Geometry check sheet. Reference: the model listing, model coordinates, mm. Face numbers are marked on the shaded views. Give positions to 0.01 mm unless a question says otherwise; leave off trailing zeros. Order: outer loops, then holes, each group sorted by start corner. A loop starts at its lowest first (then second) coordinate and runs counter-clockwise, first axis right, second up.
```python
from build123d import *

# Parameters (mm, degrees)
F1_DEPTH = 8
F2_D     = 15
F3_D     = 15
F5_W     = 30
F5_H     = 4
F6_DEPTH = 30.001


with BuildPart() as f1:
    # F0 (on Front) → F1 (new body)
    with BuildSketch(Plane.XZ):
        with BuildLine():
            Line((110, 15), (0, 15))
            ThreePointArc((0, 15), (-15, 0), (0, -15))
            Line((0, -15), (110, -15))
            ThreePointArc((110, -15), (125, 0), (110, 15))
        make_face()
    extrude(amount=F1_DEPTH)

    # F2 (through all)
    with Locations(Plane(origin=(0, 0, 0), x_dir=(1, 0, 0), z_dir=(0, 1, 0))):
        with Locations((0, 0)):
            Hole(F2_D / 2)

    # F3 (through all)
    with Locations(Plane(origin=(0, 0, 0), x_dir=(1, 0, 0), z_dir=(0, 1, 0))):
        with Locations((110, 0)):
            Hole(F3_D / 2)

    # F5 (on offset) → F6 (cut, through all)
    with BuildSketch(Plane.XY.offset(15)):
        with Locations((0, -4.0625976841)):
            Rectangle(F5_W, F5_H)
    extrude(amount=-F6_DEPTH, mode=Mode.SUBTRACT)


solid = f1.part
```
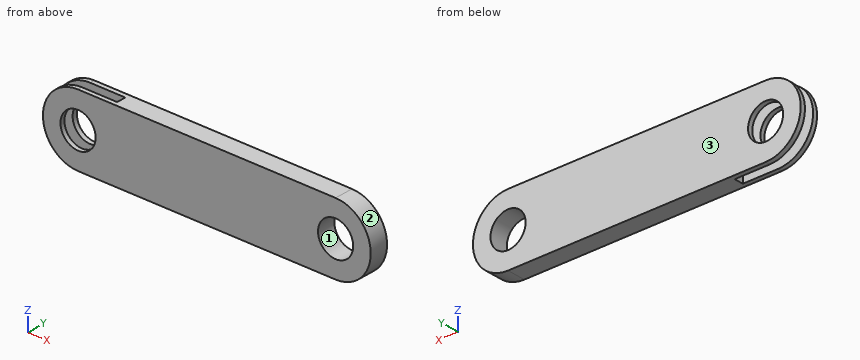
Q1. Gauge pin test, flat ends, axial feed: P1, Ø1.2, axis at y = -4, z = -7, coming from the -X side; P2, Ø9, axis at x = 1.5, z = -2, coming from the +Y side; P3, Ø1, axis at y = -1, z = -8.5, coming from the +X side. Record the tip position at first contact, or that the pin passes through.
Q2. Thickness scan on L1, parallel to Z at x = 110, y = -5.75; L2, parallel to X at y = -7.25, z = -13; L3, parallel to X at y = -4.75, z = 5. Record the ranges inside material, lowest first.
Q3. Cross-section at B-B, the plane z = 12.5. Record the boundary of the cut face in (x, y), and give its area (4 significant figures).
Q4. Release check for a two-part mould opening along Z. For the marked faces 1, 2 and 3 record: pulls with the +Z half, pulls with the -Z half, needs draft (parallel to the pull), parting line crosses it, or undercut.
Q5. Cross-section at A-A, the plane x = -6. Record the boundary of the cut face in (y, z).
Answers follow:
1. P1: stops at x = 15
1. P2: passes through
1. P3: stops at x = 122.69
2. L1: z = -15 to -7.5, 7.5 to 15
2. L2: x = -7.48 to 117.48
2. L3: x = 15 to 104.41, 115.59 to 124.14
3. outline: (-8.29, -8) - (118.29, -8) - (118.29, 0) - (-8.29, 0) - (-8.29, -2.06) - (15, -2.06) - (15, -6.06) - (-8.29, -6.06) - close
3. area: 919.5 mm2
4. face 1: undercut
4. face 2: parting line crosses it
4. face 3: needs draft
5. outline: (-8, -13.75) - (-6.06, -13.75) - (-6.06, -4.5) - (-8, -4.5) - close; (-8, 4.5) - (-6.06, 4.5) - (-6.06, 13.75) - (-8, 13.75) - close; (-2.06, -13.75) - (0, -13.75) - (0, -4.5) - (-2.06, -4.5) - close; (-2.06, 4.5) - (0, 4.5) - (0, 13.75) - (-2.06, 13.75) - close
